Read the model definition and answer for the solid it produces. Units are mm, in the model's axes. Face numbers are marked on the shaded views. A direction names the side the tool comes from. Coordinates: 2 decimals unless noted, no trailing zeros. Write each loop counter-clockwise with the first axis right and the second up, starting at its lowest first coordinate (ties: lowest second). Pieces come first, ordered by that corner, then holes.
(1) Which of the six approach directions +Z, -Z, +X, -X, +Y, -Y give full straight-line access (tool end or side, diameter ignored) to the marked faces 1, 2, 3, 4 and 5?
(2) Section A-A on x = 40.5 is taken. Write down the section's boundary in (y, z).
(3) Given pin 1 (10 mm diameter, centred on y = -6, z = -43.5, fed in from -X); pin 2 (10 mm diameter, centred on y = 1.5, z = -24, fed in from -X); pin 3 (2 mm diameter, centred on y = 7.5, z = -34.5, fed in from +X); pin 4 (2 mm diameter, centred on x = 9.5, z = -21, fed in from +Y), each flat-ended and moving along its own axis, determine where each tip first touches the part or whether it passes through.
(4) Section C-C on z = -37 is taken. Write down the section's boundary in (x, y).
(5) Find the intervals of material crossed by probe 1 along Z at (x, y) = (-25, 3); probe 2 along X at (y, z) = (14, -91.5); probe 3 along Y at (x, z) = (21, -16), in increasing order.
(6) The mould has two halves that part along X. Classify the marked faces 6, 7 and 8: +X half, -X half, draft (parallel to the pull), parting line (faces both ways), or undercut.
from build123d import *

# Parameters (mm, degrees)
BOSS_EXTRUDE1_DEPTH      = 13.5
BOSS_EXTRUDE1_DEPTH_BACK = 13.5
BOSS_EXTRUDE2_START      = -30
BOSS_EXTRUDE2_DEPTH      = 10
FILLET3_R                = 2
BOSS_EXTRUDE3_DEPTH      = 38
FILLET4_R                = 5
FILLET5_R                = 5


with BuildPart() as part:
    # Sketch1 → Boss-Extrude1 (new, two sides: drawn at the far end of the back side and taken through both)
    with BuildSketch(Plane(origin=(0, 0, 0), x_dir=(1, 0, 0), z_dir=(0, 1, 0)).offset(-BOSS_EXTRUDE1_DEPTH_BACK)):
        with BuildLine():
            Line((0, 0), (46, 0))
            ThreePointArc((46, 0), (51.656854249, 2.343145751), (54, 8))
            Line((54, 8), (54, 68))
            Line((54, 68), (26, 68))
            Line((26, 68), (26, 35))
            ThreePointArc((26, 35), (24.535533906, 31.464466094), (21, 30))
            Line((21, 30), (0, 30))
            Line((0, 30), (0, 15))
            Line((0, 15), (0, 0))
        make_face()
    extrude(amount=BOSS_EXTRUDE1_DEPTH + BOSS_EXTRUDE1_DEPTH_BACK)

    # Sketch2 → Boss-Extrude2 (add)
    with BuildSketch(Plane.XY.offset(BOSS_EXTRUDE2_START)):
        with BuildLine():
            Line((0, -13.5), (-31.5, -13.5))
            ThreePointArc((-31.5, -13.5), (-43.351405537, 2.974190082), (-23.964041865, 8.972930111))
            ThreePointArc((-23.964041865, 8.972930111), (-22.539334644, 8.22153994), (-20.949658611, 7.962102155))
            Line((-20.949658611, 7.962102155), (0, 7.962102155))
            Line((0, 7.962102155), (0, -13.5))
        make_face()
    extrude(amount=BOSS_EXTRUDE2_DEPTH)

    # Fillet3
    fillet3_edges = [part.edges().sort_by_distance(p)[0] for p in [
        (0, 7.962102155, -25),
        (0, -2.768948923, -20),
    ]]
    fillet(fillet3_edges, radius=FILLET3_R)

    # Sketch4 → Boss-Extrude3 (add)
    with BuildSketch(Plane.ZY.offset(-26)):
        with BuildLine():
            ThreePointArc((-90, 15.5), (-105.482977781, -0.726222431), (-88.549150224, -15.431948514))
            Line((-88.549150224, -15.431948514), (-68, -13.5))
            Line((-68, -13.5), (-68, 13.5))
            Line((-68, 13.5), (-87.204918033, 15.245901639))
            Line((-87.204918033, 15.245901639), (-90, 15.5))
        make_face()
    extrude(amount=-BOSS_EXTRUDE3_DEPTH)

    # Fillet4
    fillet4_edges = [part.edges().sort_by_distance(p)[0] for p in [
        (54, 0, -68),
    ]]
    fillet(fillet4_edges, radius=FILLET4_R)

    # Fillet5
    fillet5_edges = [part.edges().sort_by_distance(p)[0] for p in [
        (64, 0, -68),
    ]]
    fillet(fillet5_edges, radius=FILLET5_R - 0.0001)  # a hair under: the kernel refuses the full size


solid = part.part
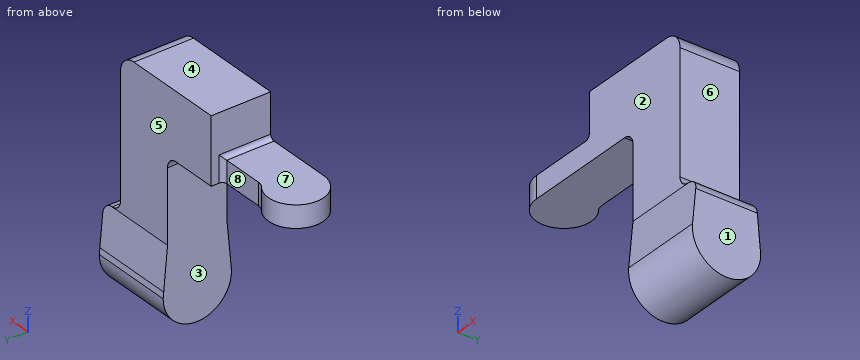
Response:
1. face 1: +Z, -Z, +X, +Y, -Y
1. face 2: +Z, +X, -X, -Y
1. face 3: -Z, -X, +Y, -Y
1. face 4: +Z, +X, -X, +Y, -Y
1. face 5: +Z, +X, -X, +Y
2. outline: (-15.43, -88.55) arc R15.5 ccw (long way) to (15.5, -90) - (13.5, -68) - (13.5, 0) - (-13.5, 0) - (-13.5, -68) - close
3. pin 1: stops at x = 26
3. pin 2: stops at x = -44
3. pin 3: stops at x = 54
3. pin 4: stops at y = 13.5
4. outline: (26, -13.5) - (54, -13.5) - (54, 13.5) - (26, 13.5) - close
5. probe 1: z = -30 to -20
5. probe 2: x = 26 to 64
5. probe 3: y = -13.5 to 13.5
6. face 6: +X half
6. face 7: draft
6. face 8: undercut
